from build123d import *

# Parameters (mm, degrees)
F0_W     = 10
F0_H     = 10
F0_R     = 22.5
F0_W_2   = 0.0176012516
F0_H_2   = 0.0236101449
F0_W_3   = 0.002938509
F0_H_3   = 0.0060267746
F1_DEPTH = 20


with BuildPart() as f1:
    # F0 (on Front) → F1 (new body)
    with BuildSketch(Plane.XZ):
        with Locations((-25, 45)):
            Rectangle(F0_W, F0_H)
        with Locations((-35, 35)):
            Rectangle(F0_W, F0_H)
        Polygon((20, 50), (-20, 50), (-20, 40), (-30, 40), (-30, 30), (-40, 30), (-40, 20), (-50, 20), (-50, -20), (-40, -20), (-40, -30), (-30, -30), (-30, -40), (-20, -40), (-20, -50), (20, -50), (20, -40), (30, -40), (30, -30), (40, -30), (40, -20), (50, -20), (50, 20), (40, 20), (40, 30), (30, 30), (30, 40), (20, 40), align=None)
        Circle(F0_R, mode=Mode.SUBTRACT)
        with Locations((-45, 25)):
            Rectangle(F0_W, F0_H)
        with Locations((25, 45)):
            Rectangle(F0_W, F0_H)
        Polygon((39.9823987484, 40), (30, 40), (30, 30), (40, 30), (40, 39.9763898551), (39.9823987484, 39.9763898551), align=None)
        with Locations((-45, -25)):
            Rectangle(F0_W, F0_H)
        with Locations((39.9911993742, 39.9881949276)):
            Rectangle(F0_W_2, F0_H_2)
        with Locations((45, 25)):
            Rectangle(F0_W, F0_H)
        with Locations((-35, -35)):
            Rectangle(F0_W, F0_H)
        with Locations((-25, -45)):
            Rectangle(F0_W, F0_H)
        with Locations((45, -25)):
            Rectangle(F0_W, F0_H)
        Polygon((40, -39.9939732254), (40, -30), (30, -30), (30, -40), (39.9823987484, -40), (39.997061491, -40), (39.997061491, -39.9939732254), align=None)
        with Locations((25, -45)):
            Rectangle(F0_W, F0_H)
        with Locations((39.9985307455, -39.9969866127)):
            Rectangle(F0_W_3, F0_H_3)
    extrude(amount=F1_DEPTH)


solid = f1.part
Verification items for the finished model (mm, model axes). A direction names the side the tool comes from. Coordinates: 2 decimals unless noted, no trailing zeros. Order: outer loops, then holes, each group sorted by start corner. A loop starts at its lowest first (then second) coordinate and runs counter-clockwise, first axis right, second up. Notation, with made-up numbers: M 42,-34 L 98,-34 A24 ccw 98,-2 Z; hole C 77,-36.75 d3. An arc over 180 degrees is marked long. One line per item, written item: value. Start each with the question number.
Item 1: Gauge pin test, flat ends, axial feed: pin 1 (11 mm diameter, centred on y = -6, z = -46.5, fed in from +X); pin 2 (10 mm diameter, centred on x = -34.5, z = 20, fed in from +Y); pin 3 (3 mm diameter, centred on x = 46.5, y = -14.5, fed in from +Z); pin 4 (11 mm diameter, centred on x = -44.5, y = -10.5, fed in from +Z). Record the tip position at first contact, or that the pin passes through.
Item 2: Sectioned sample at D-D (z = -36). Enter the section's corners in (x, y).
Item 3: Sectioned sample at A-A (z = 0). Enter the section's corners in (x, y), then the cut area to 3 significant figures.
Item 4: Access from +Z, -Z, +X, -X, +Y, -Y to the whole of each face (thin tool, end or side, straight path). Record for faces 1 (the flat face through (-30, -10, -45)), 2 (the flat face through (-30, -10, 45)), 3 (the flat face through (35, -10, 40)), 4 (the flat face through (45, -10, -30)).
Item 5: Scan lines: probe 1 along Z at (x, y) = (0, -12); probe 2 along Z at (x, y) = (-42, -13.5). Record each from-to range of solid material in increasing order.
Item 6: Sectioned sample at B-B (x = 0). Enter the section's corners in (y, z), then the cut area to 3 significant figures.
Item 7: Sectioned sample at C-C (y = -16). Enter the section's corners in (x, z).
Conclusion:
1. pin 1: stops at x = 30
1. pin 2: stops at y = 0
1. pin 3: stops at z = 30
1. pin 4: stops at z = 40
2. outline: M -40,-20 L 40,-20 L 40,0 L -40,0 Z
3. outline: M -50,-20 L -22.5,-20 L -22.5,0 L -50,0 Z; M 22.5,-20 L 50,-20 L 50,0 L 22.5,0 Z
3. area: 1,100 mm^2
4. face 1: -Z, -X, +Y, -Y
4. face 2: +Z, -X, +Y, -Y
4. face 3: +Z, +X, +Y, -Y
4. face 4: -Z, +X, +Y, -Y
5. probe 1: z = -50 to -22.5, 22.5 to 50
5. probe 2: z = -30 to 30
6. outline: M -20,-50 L 0,-50 L 0,-22.5 L -20,-22.5 Z; M -20,22.5 L 0,22.5 L 0,50 L -20,50 Z
6. area: 1,100 mm^2
7. outline: M -50,-30 L -40,-30 L -40,-40 L -30,-40 L -30,-50 L 30,-50 L 30,-40 L 40,-40 L 40,-30 L 50,-30 L 50,30 L 40,30 L 40,40 L 30,40 L 30,50 L -30,50 L -30,40 L -40,40 L -40,30 L -50,30 Z; hole C 0,0 d45
